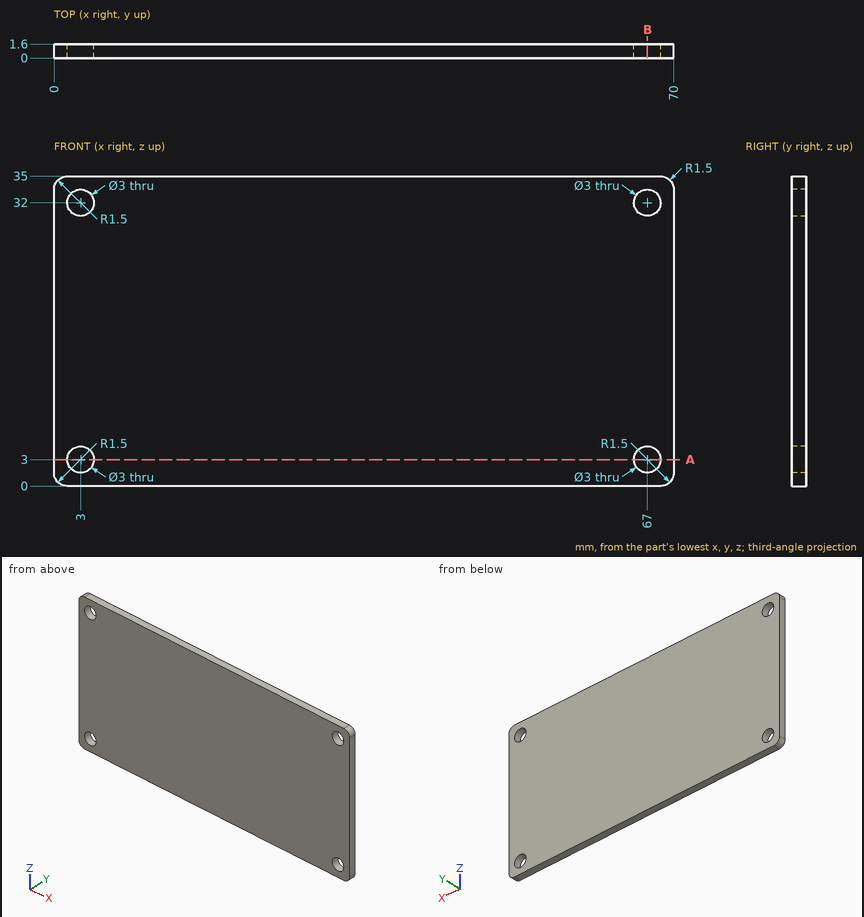
Geometry check sheet. Reference: drawing and pictorial views, mm from the part's lowest x, y, z. Give positions to 0.01 mm unless a question says otherwise; leave off trailing zeros. Order: outer loops, then holes, each group sorted by start corner. A loop starts at its lowest first (then second) coordinate and runs counter-clockwise, first axis right, second up. Notation, with made-up numbers: M 7,69 L 63,69 A30 ccw 63,98 Z; hole C 75,35 d7. An arc over 180 degrees is marked long. Answer in a Markdown table with one row per item. Add a question column.
Item 1: Section check A-A, the plane z = 3. Enter the section's corners in (x, y).
Item 2: Scan lines: probe 1 along X at (y, z) = (1, 3); probe 2 along X at (y, z) = (1.35, 31.5); probe 3 along X at (y, z) = (1, 1). Record each from-to range of solid material in increasing order. Write a range as from..to.
Item 3: Gauge pin test, flat ends, axial feed: pin 1 (1.8 mm diameter, centred on x = 3, z = 3, fed in from -Y); pin 2 (4 mm diameter, centred on x = 3, z = 32, fed in from +Y). Record the tip position at first contact, or that the pin passes through.
Item 4: Section check B-B, the plane x = 67. Enter the section's corners in (y, z), and give its area (3 significant figures).
Filled sheet:
| question | item | result |
|---|---|---|
| 1 | outline | M 0,0 L 1.5,0 L 1.5,1.6 L 0,1.6 Z; M 4.5,0 L 65.5,0 L 65.5,1.6 L 4.5,1.6 Z; M 68.5,0 L 70,0 L 70,1.6 L 68.5,1.6 Z |
| 2 | probe 1 | x = 0..1.5, 4.5..65.5, 68.5..70 |
| 2 | probe 2 | x = 0..1.59, 4.41..65.59, 68.41..70 |
| 2 | probe 3 | x = 0.09..69.91 |
| 3 | pin 1 | passes through |
| 3 | pin 2 | stops at y = 1.6 |
| 4 | outline | M 0,0 L 1.6,0 L 1.6,1.5 L 0,1.5 Z; M 0,4.5 L 1.6,4.5 L 1.6,30.5 L 0,30.5 Z; M 0,33.5 L 1.6,33.5 L 1.6,35 L 0,35 Z |
| 4 | area | 46.4 mm^2 |
